from build123d import *

# Parameters (mm, degrees)
COQUE_T       = -0.9
BOSSAGE_DEPTH = 14
ESQUISSE3_R   = 2.5
ENLEV_DEPTH   = 50.157908825


with BuildPart() as part:
    # esquisse → revolution (revolve)
    with BuildSketch(Plane.XY, mode=Mode.PRIVATE) as revolution_sk:
        Polygon((0, 0), (7.5, 0), (4, 3), (4, 5.897032863), (7.5, 5.897032863), (4, 8.897032863), (4, 12), (7.5, 12), (4, 15), (6, 24), (6, 34), (0, 34), align=None)
    revolve(revolution_sk.sketch.rotate(Axis((0, 34, 0), (0, -1, 0)), 180), axis=Axis((0, 34, 0), (0, -1, 0)))

    # coque
    coque_openings = [part.faces().sort_by_distance(p)[0] for p in [
        (0, 0, 0),
    ]]
    offset(amount=COQUE_T, openings=coque_openings, kind=Kind.INTERSECTION)

    # Esboço2 → bossage (add)
    with BuildSketch(Plane(origin=(0, 34, 0), x_dir=(1, 0, 0), z_dir=(0, 1, 0))):
        Polygon((3.499984176, 5.979139634), (-3.428094728, 6.020645027), (-6.928078904, 0.041505392), (-3.499984176, -5.979139634), (3.428094728, -6.020645027), (6.928078904, -0.041505392), align=None)
    extrude(amount=BOSSAGE_DEPTH)

    # esquisse3 → enlev (cut, through all)
    with BuildSketch(Plane(origin=(0, 48, 0), x_dir=(1, 0, 0), z_dir=(0, 1, 0))):
        with Locations(Location((0, 0, 0), (0, 0, 270))):
            Circle(ESQUISSE3_R)
    extrude(amount=-ENLEV_DEPTH, mode=Mode.SUBTRACT)


solid = part.part
Could you check a few things on this model? Use its own coordinates, in mm. A direction names the side the tool comes from. Coordinates: 2 decimals unless noted, no trailing zeros. Order: outer loops, then holes, each group sorted by start corner. A loop starts at its lowest first (then second) coordinate and runs counter-clockwise, first axis right, second up.
Q1. Will these pins go through, and if not, where does the flat tip stop? pin 1 (4.5 mm diameter, centred on x = 0, z = 0, fed in from -Y); pin 2 (8 mm diameter, centred on x = -2, z = 3, fed in from -Y); pin 3 (6 mm diameter, centred on y = 31, z = -5.5, fed in from -X); pin 4 (4.5 mm diameter, centred on x = 0.5, z = 3.5, fed in from -Y).
Q2. Thinking about a two-plate mould opening in Y: for faces 4 (the cylindrical face through (-2.957, 4.721, -0.931)), 5 (the flat face through (-3, 0, 6)), 6 (the flat face through (-0.1, 12.9, 3.3)), 7 (the cylindrical face through (-4.864, 28.662, -1.532)), which applies, released by +Y, released by -Y, zero draft, split by the parting line, or undercut?
Q3. Suppose I cut it at C-C on y = 18. Please give me the cut outline in (x, z).
Q4. Which directions (+Z, -Z, +X, -X, +Y, -Y) give clear straight access to the entire face, cutting with the end or side of a thin tool? Please do faces 1 (the cylindrical face through (-5.723, 29.07, -1.802)), 2 (the flat face through (2.95, 34, 5.4)), 3 (the flat face through (5.154, 40.902, 3.073)).
Q5. Please list where these lines run through material, in increasing order: L1, parallel to Z at x = 0, y = 29; L2, parallel to Y at x = 6.25, z = 3; L3, parallel to Z at x = -1.25, y = 32.5.
Q6. Suppose I cut it at A-A on y = 36. Please give me the cut outline in (x, z).
Q7. Suppose I cut it at B-B on y = 8. Please give me the cut outline in (x, z).
Answer:
1. pin 1: passes through
1. pin 2: stops at y = 0
1. pin 3: stops at x = -5.45
1. pin 4: stops at y = 0.28
2. face 4: zero draft
2. face 5: released by -Y
2. face 6: undercut
2. face 7: undercut
3. outline: circle Ø9.33 at (0, 0); hole circle Ø7.49 at (0, 0)
4. face 1: none
4. face 2: +Z, +X
4. face 3: +Z, +X, +Y
5. L1: z = -6 to -5.1, 5.1 to 6
5. L2: y = 0 to 0.49, 5.9 to 6.38, 12 to 12.49
5. L3: z = -5.87 to -4.94, 4.94 to 5.87
6. outline: (-6.93, -0.04) - (-3.43, -6.02) - (3.5, -5.98) - (6.93, 0.04) - (3.43, 6.02) - (-3.5, 5.98) - close; hole circle Ø5 at (0, 0)
7. outline: circle Ø10.09 at (0, 0); hole circle Ø7.33 at (0, 0)
